Here's the drawing with two shaded views (mm, measured from the low corner). I have some questions. Give positions to 0.01 mm unless a question says otherwise; leave off trailing zeros. Write each loop counter-clockwise with the first axis right and the second up, starting at its lowest first coordinate (ties: lowest second). Pieces come first, ordered by that corner, then holes. Notation, with made-up numbers: (72.25, 55) -> (82.25, 55) arc R18 cw to (82.25, 69) -> close; hole circle Ø10 at (17.5, 66). An arc over 180 degrees is marked (long way). One line per item, written item: value.
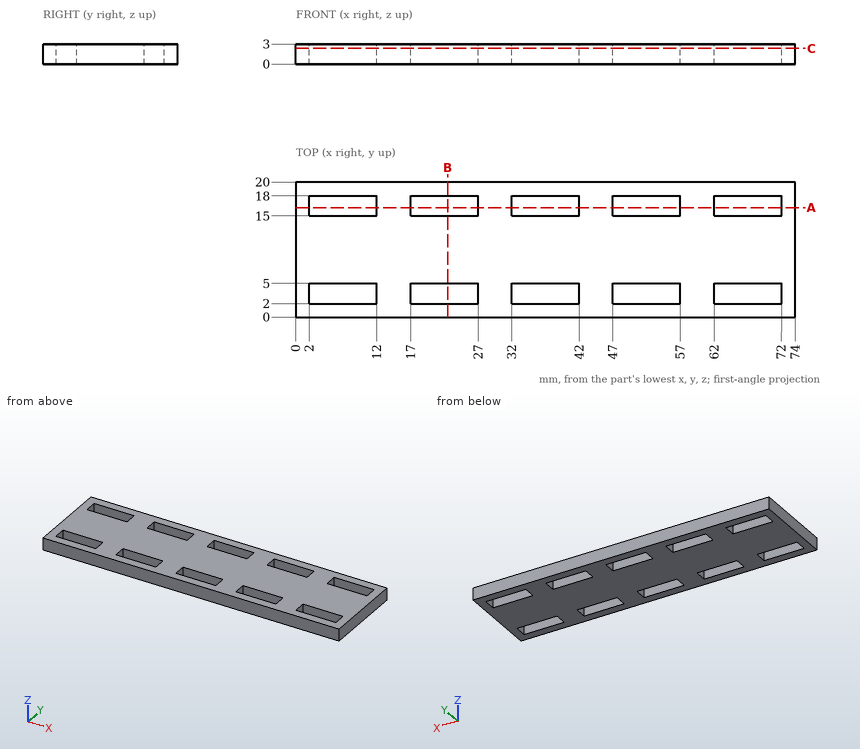
1) I need wall thicknesses on L1, parallel to X at y = 15.5, z = 1.35; L2, parallel to Y at x = 55.5, z = 2.5. Which ranges of each line are inside material? Lowest first, please.
Answer list:
L1: x = 0 to 2, 12 to 17, 27 to 32, 42 to 47, 57 to 62, 72 to 74
L2: y = 0 to 2, 5 to 15, 18 to 20
2) If we section it at C-C (z = 2.35): State how many separate pieces and enclosed holes the cut face has, and give its area (3 significant figures).
Answer list:
separate pieces: 1
enclosed holes: 10
area: 1,180 mm^2
3) If we section it at A-A (y = 16.25): Write out the boundary of the cut face in (x, z), and give its area (3 significant figures).
Answer list:
outline: (0, 0) -> (2, 0) -> (2, 3) -> (0, 3) -> close; (12, 0) -> (17, 0) -> (17, 3) -> (12, 3) -> close; (27, 0) -> (32, 0) -> (32, 3) -> (27, 3) -> close; (42, 0) -> (47, 0) -> (47, 3) -> (42, 3) -> close; (57, 0) -> (62, 0) -> (62, 3) -> (57, 3) -> close; (72, 0) -> (74, 0) -> (74, 3) -> (72, 3) -> close
area: 72.0 mm^2
4) If we section it at B-B (x = 22.5): Write out the boundary of the cut face in (y, z).
Answer list:
outline: (0, 0) -> (2, 0) -> (2, 3) -> (0, 3) -> close; (5, 0) -> (15, 0) -> (15, 3) -> (5, 3) -> close; (18, 0) -> (20, 0) -> (20, 3) -> (18, 3) -> close
5) Will this pin go through, and if not, where does the flat tip stop? pin 1 (1.5 mm diameter, centred on y = 3.5, z = 1, fed in from -X).
Answer list:
pin 1: stops at x = 0
